Design review of the part built by this model. Coordinates are the model's own, in mm. Face numbers are marked on the shaded views. A direction names the side the tool comes from. Give positions to 0.01 mm unless a question says otherwise; leave off trailing zeros. Order: outer loops, then holes, each group sorted by start corner. A loop starts at its lowest first (then second) coordinate and runs counter-clockwise, first axis right, second up. Notation, with made-up numbers: (73, 15.25) -> (107, 15.25) arc R9 cw to (107, 31.25) -> close; hole circle Ø2 at (-9.75, -29). An arc over 180 degrees is marked (long way). One line per item, written item: value.
from build123d import *

# Parameters (mm, degrees)
F0_W     = 16
F0_H     = 8
F1_DEPTH = 9.6
F2_W     = 12.8
F2_H     = 4.8
F2_R     = 1.6
F3_DEPTH = 8
F4_R     = 2.4
F5_DEPTH = 1.6
F6_R     = 1.2
F7_DEPTH = 1.6


with BuildPart() as f1:
    # F0 (on Top) → F1 (new body)
    with BuildSketch(Plane.XY):
        Rectangle(F0_W, F0_H)
    extrude(amount=F1_DEPTH)

    # F2 (on face) → F3 (cut)
    with BuildSketch(Plane(origin=(0, 0, 0), x_dir=(1, 0, 0), z_dir=(0, 0, -1))):
        Rectangle(F2_W, F2_H)
        Circle(F2_R, mode=Mode.SUBTRACT)
    extrude(amount=-F3_DEPTH, mode=Mode.SUBTRACT)

    # F4 (on face) → F5 (join)
    with BuildSketch(Plane.XY.offset(9.6)):
        with Locations((-4, 0)):
            Circle(F4_R)
        with Locations((4, 0)):
            Circle(F4_R)
    extrude(amount=F5_DEPTH)

    # F6 (on face) → F7 (cut)
    with BuildSketch(Plane(origin=(0, 0, 8), x_dir=(1, 0, 0), z_dir=(0, 0, -1))):
        with Locations((4, 0)):
            Circle(F6_R)
        with Locations((-4, 0)):
            Circle(F6_R)
    extrude(amount=-F7_DEPTH, mode=Mode.SUBTRACT)


solid = f1.part
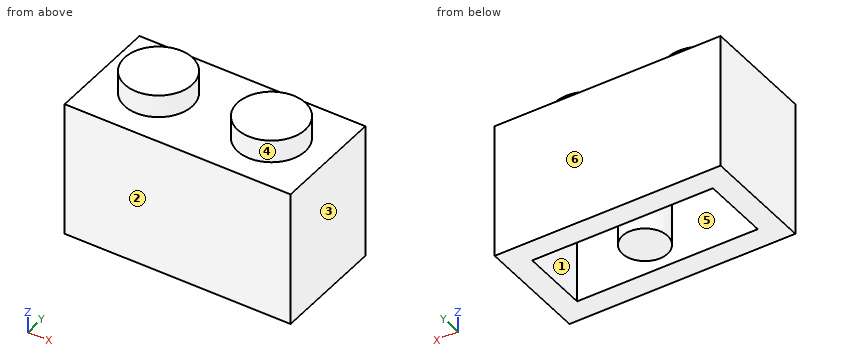
Item 1: To check wall thickness, follow line 1 along X through (y, z) = (0, 8.45); line 2 along Y through (x, z) = (-0.75, 5.5); line 3 along Y through (x, z) = (3.25, 6.25). State the ranges of each line that lie inside material, in increasing order. Write a range as from..to.
Returned:
line 1: -8..-5.2, -2.8..2.8, 5.2..8
line 2: -4..-2.4, -1.41..1.41, 2.4..4
line 3: -4..-2.4, 2.4..4
Item 2: Machinability: for the marked faces 4, 5 and 6, which of the approach directions +Z, -Z, +X, -X, +Y, -Y give a long, thin tool a straight path to every point of the face, cutting with its end or side? Answer none if there is none.
Returned:
face 4: +Z
face 5: -Z
face 6: +Z, -Z, +X, -X, +Y
Item 3: Draft analysis for pull direction X (two halves, no side actions). For the marked faces 1, 2 and 3, state which applies: pulls with the +X half, pulls with the -X half, needs draft (parallel to the pull), parting line crosses it, or undercut.
Returned:
face 1: undercut
face 2: needs draft
face 3: pulls with the +X half
Item 4: Clearance check with flat-ended pins moving along their axes: P1, Ø1.2, axis at x = -4.5, y = 0, coming from the -Z side; P2, Ø2.5, axis at x = 3.5, y = -0.5, coming from the -Z side. State where each tip first meets the part, or that it passes through.
Returned:
P1: z = 9.6
P2: z = 8
Item 5: Add section A-A on z = 6. Give the boundary of the cut face in (x, y).
Returned:
outline: (-8, -4) -> (8, -4) -> (8, 4) -> (-8, 4) -> close; circle Ø3.2 at (0, 0); hole (-6.4, -2.4) -> (6.4, -2.4) -> (6.4, 2.4) -> (-6.4, 2.4) -> close
Item 6: Add section D-D on x = 4. Give the boundary of the cut face in (y, z), plus the area to 3 significant figures.
Returned:
outline: (-4, 0) -> (-2.4, 0) -> (-2.4, 8) -> (-1.2, 8) -> (-1.2, 9.6) -> (1.2, 9.6) -> (1.2, 8) -> (2.4, 8) -> (2.4, 0) -> (4, 0) -> (4, 9.6) -> (2.4, 9.6) -> (2.4, 11.2) -> (-2.4, 11.2) -> (-2.4, 9.6) -> (-4, 9.6) -> close
area: 42.2 mm²
Item 7: Add section B-B on x = 0. Give the boundary of the cut face in (y, z).
Returned:
outline: (-4, 0) -> (-2.4, 0) -> (-2.4, 8) -> (-1.6, 8) -> (-1.6, 0) -> (1.6, 0) -> (1.6, 8) -> (2.4, 8) -> (2.4, 0) -> (4, 0) -> (4, 9.6) -> (-4, 9.6) -> close
Item 8: Add section C-C on y = 0. Give the boundary of the cut face in (x, z), plus the area to 3 significant figures.
Returned:
outline: (-8, 0) -> (-6.4, 0) -> (-6.4, 8) -> (-5.2, 8) -> (-5.2, 9.6) -> (-2.8, 9.6) -> (-2.8, 8) -> (-1.6, 8) -> (-1.6, 0) -> (1.6, 0) -> (1.6, 8) -> (2.8, 8) -> (2.8, 9.6) -> (5.2, 9.6) -> (5.2, 8) -> (6.4, 8) -> (6.4, 0) -> (8, 0) -> (8, 9.6) -> (6.4, 9.6) -> (6.4, 11.2) -> (1.6, 11.2) -> (1.6, 9.6) -> (-1.6, 9.6) -> (-1.6, 11.2) -> (-6.4, 11.2) -> (-6.4, 9.6) -> (-8, 9.6) -> close
area: 84.5 mm²
